Input: dimensioned drawing with shaded views. Units: mm. Origin: part minimum x, y, z. Round coordinates to 2 decimals unless told otherwise and drop trailing zeros. Loops run counter-clockwise (first coordinate to the right, second up) from the corner with the lowest first, then second, coordinate; pieces in that order, holes last. Notation, with made-up numbers: (21.25, 55) -> (40.25, 55) arc R15 ccw to (40.25, 59) -> close; hole circle Ø1 at (65, 29.25). An arc over 180 degrees is marked (long way). Answer as a JSON object with one key per item and string values.
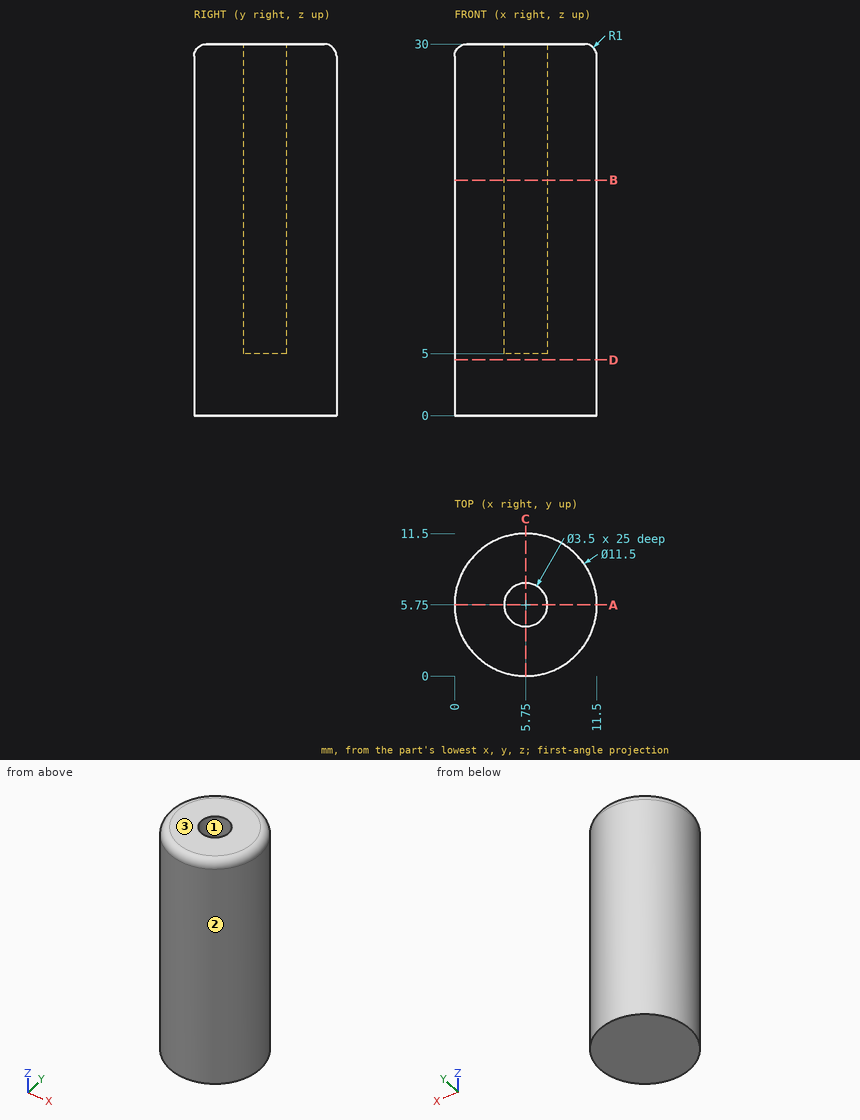
1) Section D-D, the plane z = 4.5. Output: boundary loops of the cut face in (x, y), plus the area to 3 significant figures.
Output:
{"outline": "circle Ø11.5 at (5.75, 5.75)", "area": "104 mm^2"}
2) Ray query, probe 1 along Y at (x, z) = (5.75, 15.75); probe 2 along Z at (x, y) = (5, 7); probe 3 along X at (y, z) = (5, 23.5). Return the intervals inside material, ascending.
Output:
{"probe 1": "y = 0 to 4, 7.5 to 11.5", "probe 2": "z = 0 to 5", "probe 3": "x = 0.05 to 4.17, 7.33 to 11.45"}
3) Draft query along Y for the marked faces 1, 2 and 3. Return one class per face: +Y half, -Y half, draft (parallel to the pull), parting line (faces both ways), or undercut.
Output:
{"face 1": "undercut", "face 2": "parting line", "face 3": "draft"}
4) Contact query for a flat-ended pin moving along its axis: P1, Ø3, axis at y = 10, z = 9, coming from the +X side. Output: stop coordinate, or through.
Output:
{"P1": "stops at x = 10.8"}
5) Section A-A, the plane y = 5.75. Output: boundary loops of the cut face in (x, z), plus the area to 3 significant figures.
Output:
{"outline": "(0, 0) -> (11.5, 0) -> (11.5, 29) arc R1 ccw to (10.5, 30) -> (7.5, 30) -> (7.5, 5) -> (4, 5) -> (4, 30) -> (1, 30) arc R1 ccw to (0, 29) -> close", "area": "257 mm^2"}
6) Section B-B, the plane z = 19. Output: boundary loops of the cut face in (x, y).
Output:
{"outline": "circle Ø11.5 at (5.75, 5.75); hole circle Ø3.5 at (5.75, 5.75)"}
